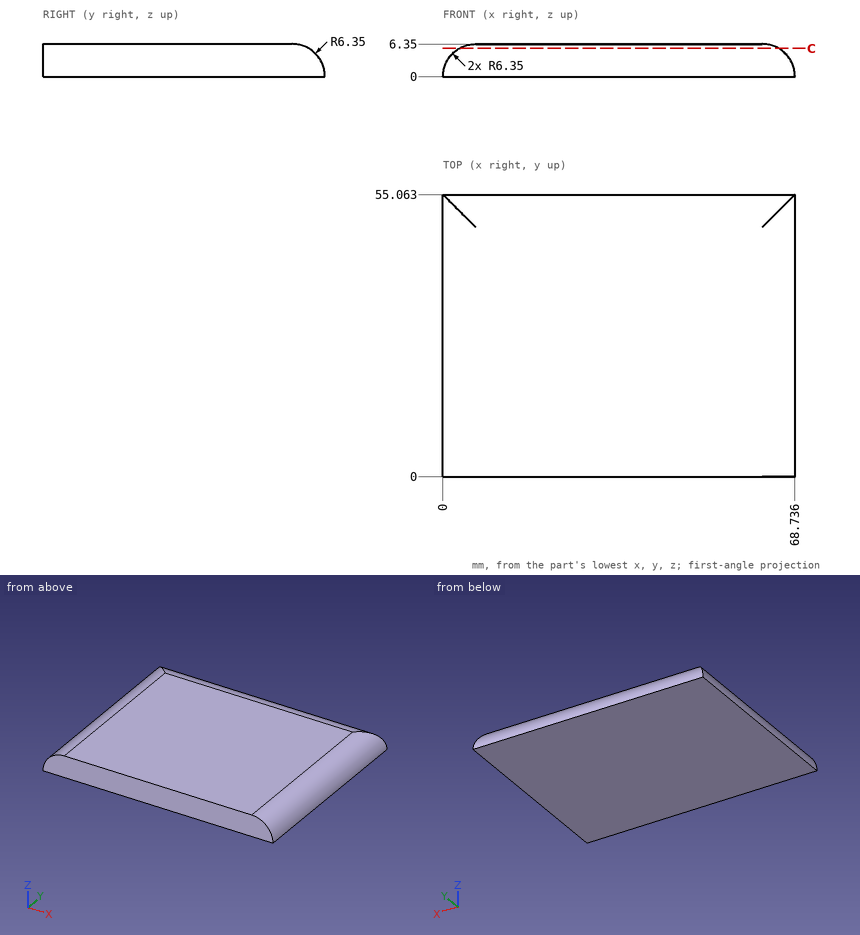
Check sheet for the drawn part. Datum: minimum x, y, z corner. Units: mm. Round coordinates to 2 decimals unless told otherwise and drop trailing zeros. Loops run counter-clockwise (first coordinate to the right, second up) from the corner with the lowest first, then second, coordinate; pieces in that order, holes last.
Item 1: Gauge pin test, flat end, axial feed: pin 1 (1.5 mm diameter, centred on y = 33, z = 4, fed in from -X) (1 decimal). Record the tip position at first contact, or that the pin passes through.
Item 2: Cross-section at C-C on z = 5.5. Record the boundary of the cut face in (x, y).
Item 3: Thickness scan on line 1 (Z direction, x = 6, y = 4.5); line 2 (X direction, y = 33, z = 4); line 3 (Y direction, x = 26, z = 2.25). Record the ranges inside material, lowest first.
Answer sheet:
1. pin 1: stops at x = 0.9
2. outline: (3.18, 0) - (65.56, 0) - (65.56, 51.89) - (3.18, 51.89) - close
3. line 1: z = 0 to 6.34
3. line 2: x = 1.42 to 67.32
3. line 3: y = 0 to 54.65
